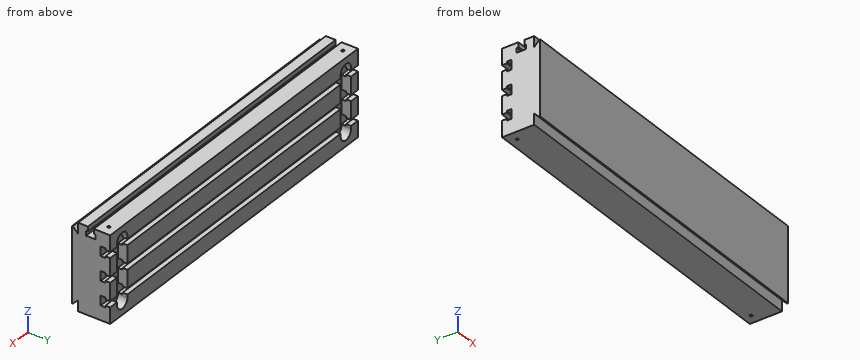
```python
from build123d import *
from OCP.BRepFilletAPI import BRepFilletAPI_MakeChamfer

# Parameters (mm, degrees)
SKETCH1_W                      = 914.4
SKETCH1_H                      = 228.6
EXTRUDE1_DEPTH                 = 85.725
CUT_EXTRUDE1_DEPTH             = 480.004285602
LPATTERN1_COUNT                = 2
LPATTERN1_PITCH                = 63.5
LPATTERN1_COL_COUNT            = 2
LPATTERN1_COL_PITCH            = 63.5
CUT_EXTRUDE2_DEPTH             = 480.004285602
CUT_EXTRUDE2_DEPTH_BACK        = 480.004285602
EXTRUDE2_DEPTH                 = 457.2
EXTRUDE2_DEPTH_BACK            = 457.2
CHAMFER1_SIZE                  = 2.54
CHAMFER1_SIZE2                 = 1.796051224
CUT_EXTRUDE3_REACH             = 484.098
M8X1_0_TAPPED_HOLE1_AT_2_COUNT = 2
M8X1_0_TAPPED_HOLE1_AT_2_PITCH = 863.6


with BuildPart() as part:
    # Sketch1 → Extrude1 (new body)
    with BuildSketch(Plane(origin=(0, 0, 0), x_dir=(1, 0, 0), z_dir=(0, 1, 0))):
        Rectangle(SKETCH1_W, SKETCH1_H)
    extrude(amount=-EXTRUDE1_DEPTH)

    # Sketch2 → Cut-Extrude1 (cut, symmetric)
    with BuildSketch(Plane(origin=(0, 0, 0), x_dir=(0, 0, -1), z_dir=(1, 0, 0))):
        Polygon((12.7, -25.4), (12.7, -12.7), (7.9375, -12.7), (7.9375, 0), (-7.9375, 0), (-7.9375, -12.7), (-12.7, -12.7), (-12.7, -25.4), align=None)
    cut_extrude1 = extrude(amount=CUT_EXTRUDE1_DEPTH, both=True, mode=Mode.SUBTRACT)

    # LPattern1: Cut-Extrude1 ×2
    with Locations(*[(0, 0, -i * LPATTERN1_PITCH) for i in range(1, LPATTERN1_COUNT)]):
        add(cut_extrude1, mode=Mode.SUBTRACT)

    # LPattern1 col: Cut-Extrude1 ×2
    with Locations(*[(0, 0, i * LPATTERN1_COL_PITCH) for i in range(1, LPATTERN1_COL_COUNT)]):
        add(cut_extrude1, mode=Mode.SUBTRACT)

    # Sketch3 → Cut-Extrude2 (cut, two sides: drawn at the far end of the back side and taken through both)
    with BuildSketch(Plane(origin=(0, 0, 0), x_dir=(0, 0, -1), z_dir=(1, 0, 0)).offset(-CUT_EXTRUDE2_DEPTH_BACK)):
        Polygon((-114.3, -59.51659036), (-101.6, -59.51659036), (-101.6, -64.27909036), (-88.9, -64.27909036), (-88.9, -38.87909036), (-101.6, -38.87909036), (-101.6, -43.64159036), (-114.3, -43.64159036), align=None)
    extrude(amount=CUT_EXTRUDE2_DEPTH + CUT_EXTRUDE2_DEPTH_BACK, mode=Mode.SUBTRACT)

    # Sketch4 → Extrude2 (add, two sides: drawn at the far end of the back side and taken through both)
    with BuildSketch(Plane(origin=(0, 0, 0), x_dir=(0, 0, -1), z_dir=(1, 0, 0)).offset(-EXTRUDE2_DEPTH_BACK)):
        Polygon((-85.725, -85.725), (-101.6, -101.6), (101.6, -101.6), (85.725, -85.725), align=None)
    extrude(amount=EXTRUDE2_DEPTH + EXTRUDE2_DEPTH_BACK)

    # Chamfer1: one chamfer whose edges measure the first distance from different faces: ONE call of the kernel's chamfer builder (chamfer() names one face for all edges)
    chamfer1_edges_1 = [part.edges().sort_by_distance(p)[0] for p in [
        (0, -101.6, -101.6),
    ]]
    chamfer1_side_1 = [part.faces().sort_by_distance(p)[0] for p in [
        (0, -101.6, 0),
    ]]
    chamfer1_edges_2 = [part.edges().sort_by_distance(p)[0] for p in [
        (0, -101.6, 101.6),
    ]]
    chamfer1_side_2 = [part.faces().sort_by_distance(p)[0] for p in [
        (0, -93.6625, 93.6625),
    ]]
    chamfer1 = BRepFilletAPI_MakeChamfer(part.part.solid().wrapped)
    for e in chamfer1_edges_1:
        chamfer1.Add(CHAMFER1_SIZE, CHAMFER1_SIZE2, e.wrapped, chamfer1_side_1[0].wrapped)  # the first distance lies on this face
    for e in chamfer1_edges_2:
        chamfer1.Add(CHAMFER1_SIZE, CHAMFER1_SIZE2, e.wrapped, chamfer1_side_2[0].wrapped)  # the first distance lies on this face
    add(Compound.cast(chamfer1.Shape()), mode=Mode.REPLACE)

    # Cut-Extrude3: up to this face of the body (flat: up to its plane)
    cut_extrude3_end = Plane(part.part.faces().sort_by_distance((0, -25.4, 63.5))[0])
    # Sketch5 → Cut-Extrude3 (cut, up to the picked face)
    with BuildSketch(Plane(origin=(0, 0, 0), x_dir=(-1, 0, 0), z_dir=(0, 1, 0)), mode=Mode.PRIVATE) as cut_extrude3_sk1:
        with BuildLine():
            Line((431.8, -79.375), (431.8, 79.375))
            ThreePointArc((431.8, 79.375), (412.75, 98.425), (393.7, 79.375))
            Line((393.7, 79.375), (393.7, -79.375))
            ThreePointArc((393.7, -79.375), (412.75, -98.425), (431.8, -79.375))
        make_face()
    cut_extrude3_tool1 = split(extrude(cut_extrude3_sk1.sketch, amount=-CUT_EXTRUDE3_REACH, mode=Mode.PRIVATE), bisect_by=cut_extrude3_end, keep=Keep.BOTH, mode=Mode.PRIVATE)
    cut_extrude3 = cut_extrude3_tool1.solids().sort_by(Axis((-412.75, 0, 0), (0, -1, 0)))[0]
    add(cut_extrude3, mode=Mode.SUBTRACT)

    # Mirror1: Cut-Extrude3 across plane
    add(cut_extrude3.mirror(Plane(origin=(0, 0, 0), x_dir=(0, 0, 1), z_dir=(1, 0, 0))), mode=Mode.SUBTRACT)

    # Sketch6 → M8x1.0 Tapped Hole1 (revolve, cut)
    with BuildSketch(Plane(origin=(431.8, -22, 114.3), x_dir=(0, -1, 0), z_dir=(1, 0, 0))):
        Polygon((0, 0), (0, 20.103001567), (3.5, 17.9999894), (3.5, 0), align=None)
    m8x1_0_tapped_hole1 = revolve(axis=Axis((431.8, -22, 120.65), (0, 0, -1)), mode=Mode.SUBTRACT)

    # M8x1.0 Tapped Hole1 at 2: M8x1.0 Tapped Hole1 ×2
    with Locations(*[(-i * M8X1_0_TAPPED_HOLE1_AT_2_PITCH, 0, 0) for i in range(1, M8X1_0_TAPPED_HOLE1_AT_2_COUNT)]):
        add(m8x1_0_tapped_hole1, mode=Mode.SUBTRACT)

    # Mirror2: M8x1.0 Tapped Hole1 across plane
    add(m8x1_0_tapped_hole1.mirror(Plane.XY), mode=Mode.SUBTRACT)

    # Mirror2 copy 1 sketch → Mirror2 copy 1 (revolve, cut)
    with BuildSketch(Plane(origin=(-431.8, -22, -114.3), x_dir=(0, -1, 0), z_dir=(1, 0, 0))):
        Polygon((0, 0), (0, -20.103001567), (3.5, -17.9999894), (3.5, 0), align=None)
    revolve(axis=Axis((-431.8, -22, -120.65), (0, 0, -1)), mode=Mode.SUBTRACT)


solid = part.part
```
Geometry: final body of the model. Coordinates: model frame, mm. Coordinates: 2 decimals unless noted, no trailing zeros. Order: outer loops, then holes, each group sorted by start corner. A loop starts at its lowest first (then second) coordinate and runs counter-clockwise, first axis right, second up. Notation, with made-up numbers: (-37.75, 29.5) -> (-11.75, 29.5) arc R10 cw to (-11.75, 47.5) -> close; hole circle Ø11 at (-3, 34). An arc over 180 degrees is marked (long way). Answer in a Markdown table with one row per item.
Item 1: Section B-B on z = 30. Output: boundary loops of the cut face in (x, y).
Return value:
| item | result |
|---|---|
| outline | (-457.2, -101.6) -> (457.2, -101.6) -> (457.2, 0) -> (431.8, 0) -> (431.8, -25.4) -> (393.7, -25.4) -> (393.7, 0) -> (-393.7, 0) -> (-393.7, -25.4) -> (-431.8, -25.4) -> (-431.8, 0) -> (-457.2, 0) -> close |
Item 2: Contact query for flat-ended pins moving along their axis: P1, Ø14.5, axis at x = 126, z = -105, coming from the -Y side; P2, Ø5, axis at x = 112.5, y = -90, coming from the +Z side. Output: stop coordinate, or through.
Return value:
| item | result |
|---|---|
| P1 | stops at y = -101.6 |
| P2 | stops at z = 92.5 |
Item 3: Section A-A on x = -412.75. Output: boundary loops of the cut face in (y, z) (3 decimals), plus the area to 3 significant figures.
Return value:
| item | result |
|---|---|
| outline | (-101.6, -99.06) -> (-100.33, -100.33) -> (-85.725, -85.725) -> (-85.725, -114.3) -> (0, -114.3) -> (0, -98.425) -> (-25.4, -98.425) -> (-25.4, 98.425) -> (0, 98.425) -> (0, 114.3) -> (-43.642, 114.3) -> (-43.642, 101.6) -> (-38.879, 101.6) -> (-38.879, 88.9) -> (-64.279, 88.9) -> (-64.279, 101.6) -> (-59.517, 101.6) -> (-59.517, 114.3) -> (-85.725, 114.3) -> (-85.725, 85.725) -> (-99.804, 99.804) -> (-101.6, 99.804) -> close |
| area | 17,000 mm² |
Item 4: Ray query, L1, parallel to X at y = -22, z = -103; L2, parallel to Z at x = -340, y = -9; L3, parallel to Y at x = 431.8, z = 103.5 (3 decimals). Return the intervals inside material, ascending.
Return value:
| item | result |
|---|---|
| L1 | x = -457.2 to -435.3, -428.3 to 428.3, 435.3 to 457.2 |
| L2 | z = -114.3 to -71.44, -55.56 to -7.94, 7.94 to 55.56, 71.44 to 114.3 |
| L3 | y = -85.725 to -59.517, -43.642 to -25.5, -18.5 to 0 |
